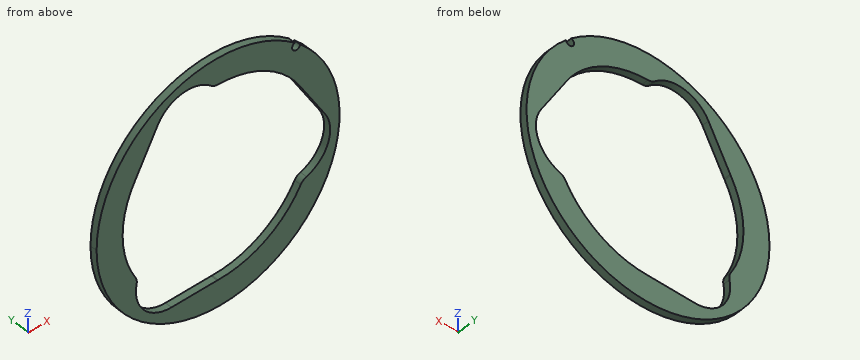
Autodesk Inventor part; units mm, degrees
ref_plane "YZ Plane" through (0, 0, 0) normal (1, 0, 0) x (0, 1, 0)
ref_plane "XZ Plane" through (0, 0, 0) normal (0, 1, 0) x (-1, 0, 0)
ref_plane "XY Plane" through (0, 0, 0) normal (0, 0, 1) x (1, 0, 0)
sketch "Sketch2" plane through (0, 0, 0) normal (0, 1, 0) x (-1, 0, 0)
  circle A0 centre (0, 0) radius 55
  circle A1 centre (0, 0) radius 70
  dimension "d18" = 110
  dimension "d19" = 140
extrude "Extrusion3" add sketch "Sketch2" along normal blind 4
sketch "Sketch3" plane through (0, 4, 0) normal (0, 1, 0) x (1, 0, 0)
  circle A0 centre (0, 0) radius 55
  circle A1 centre (0, 0) radius 70
  arc A2 (0, -55) -> (-3.9836, -56.5132) centre (0, -61) ccw
  line L0 (0, -70) -> (0, 0) construction
  line L1 (0, 0) -> (-47.6314, -27.5) construction
  circle A3 centre (0, 0) radius 65 construction
  arc A4 (-34.8476, -51.084) -> (-3.9836, -56.5132) centre (-17.2622, -41.5574) ccw
  line L2 (-34.8476, -51.084) -> (-47.3798, -27.9505)
  arc A5 (-47.3798, -27.9505) -> (-47.6411, -27.4832) centre (-64.9651, -37.4771) ccw
  dimension "d24" = 60
  dimension "d31" = 6
  dimension "d33" = 20
  dimension "d34" = 130
extrude "Extrusion4" cut sketch "Sketch3" against normal blind 6 contours A0 A2 A4 L2 A5
pattern_circular "Circular Pattern2" count 3 over 360 about axis through (0, 0, 0) along (0, 1, 0) of "Extrusion4"
sketch "Sketch4" plane through (0, 0, 0) normal (0, -1, 0) x (1, 0, 0)
  circle A0 centre (45.0297, 52.0628) radius 2.3813
  circle A1 centre (45.0297, 52.0628) radius 2.3813
extrude "Extrusion5" cut sketch "Sketch4" against normal blind 5.25
properties part number "launcher.cam"
Read the model definition and answer for the solid it produces. Units are mm, in the model's axes. Give positions to 0.01 mm unless a question says otherwise; leave off trailing zeros. Order: outer loops, then holes, each group sorted by start corner. A loop starts at its lowest first (then second) coordinate and runs counter-clockwise, first axis right, second up.
(1) Find section B-B (z = -12). Give the vertices of the cut face in (x, y).
(2) Find section C-C (y = 1). Give the vertices of the cut face in (x, z).
(3) Straight lines are drawn through the part: L1, parallel to X at y = 2.15, z = 42.5; L2, parallel to X at y = 0.9, z = 57.5; L3, parallel to Z at x = -35, y = 2.15. For each, find the intervals that lie inside material, in ascending order.
(4) Find section A-A (x = 34). Give the vertices of the cut face in (y, z), plus the area to 3 significant figures.
(5) Given pin 1 (4 mm diameter, centred on x = 45.03, z = 52.06, fed in from +Y); pin 2 (2 mm diameter, centred on x = -40, z = 52.5, fed in from -Y), each flat-ended and moving along its own axis, determine where each tip first touches the part or whether it passes through.
Result sheet:
1. outline: (-68.96, 0) - (-53.67, 0) - (-53.67, 4) - (-68.96, 4) - close; (63.65, 0) - (68.96, 0) - (68.96, 4) - (63.65, 4) - close
2. outline: (44.19, 54.29) arc R70 ccw (long way) to (47.36, 51.55) arc R2.38 cw (long way) to start; hole (-47.64, 27.48) arc R55 ccw to (-47.63, -27.5) arc R6 cw to (-46.95, -31.71) arc R20 ccw to (-26.82, -55.72) - (-0.52, -55.01) arc R20.02 cw to (0.02, -55) arc R55 ccw to (47.63, -27.5) arc R6 cw to (50.93, -24.81) arc R20 ccw to (61.66, 4.64) - (47.9, 27.06) arc R20.02 cw to (47.62, 27.52) arc R55 ccw to (0, 55) arc R6 cw to (-3.98, 56.51) arc R20 ccw to (-34.85, 51.08) - (-47.38, 27.95) arc R20.02 cw to start
3. L1: x = -55.62 to -39.5, 34.91 to 55.62
3. L2: x = -39.92 to -29.34, -5.19 to 39.92
3. L3: z = -60.62 to -54.21, 50.8 to 60.62
4. outline: (0, -61.19) - (4, -61.19) - (4, -43.23) - (0, -43.23) - close; (0, 43.23) - (4, 43.23) - (4, 61.19) - (0, 61.19) - close
4. area: 144 mm2
5. pin 1: passes through
5. pin 2: stops at y = 0
